For this review, take the finished solid that the model builds, in its own axes (mm). A direction names the side the tool comes from. Coordinates: 2 decimals unless noted, no trailing zeros.
```python
from build123d import *

# Parameters (mm, degrees)
BOSS_EXTRUDE1_DEPTH = 0.7
SCALE1_SCALE        = 3


with BuildPart() as part:
    # Sketch1 → Boss-Extrude1 (new body)
    with BuildSketch(Plane.XY):
        with BuildLine():
            add(Edge.make_bspline(
                [(1.308612852, 4.749134037), (1.089185384, 3.585197579), (1.793550911, 2.587518606)],
                knots=[0, 0, 0, 1, 1, 1], degree=2))
            ThreePointArc((1.793550911, 2.587518606), (1.734959229, -0.853049688), (-1.670369344, -0.358397807))
            Line((-1.670369344, -0.358397807), (1.14, -0.358397807))
            Line((1.14, -0.358397807), (1.14, 0))
            Line((1.14, 0), (0.84, 0))
            Line((0.84, 0), (0.84, 0.615282796))
            Line((0.84, 0.615282796), (0.34, 0.615282796))
            Line((0.34, 0.615282796), (0.34, 0))
            Line((0.34, 0), (0, 0))
            Line((0, 0), (0, 0.615282796))
            Line((0, 0.615282796), (-0.5, 0.615282796))
            Line((-0.5, 0.615282796), (-0.5, 0.015282796))
            Line((-0.5, 0.015282796), (-1.86741437, 0.015282796))
            add(Edge.make_bspline(
                [(-1.86741437, 0.015282796), (-1.967195235, 0.235858372), (-2.024440964, 0.467418027), (-2.039152584, 0.709940467)],
                knots=[0, 0, 0, 0, 0.800781106, 0.800781106, 0.800781106, 0.800781106], degree=3))
            add(Edge.make_bspline(
                [(-2.039152584, 0.709940467), (-2.047148733, 0.925627975), (-2.02218467, 1.604112941), (-1.789435207, 2.864813182), (-0.855181509, 3.674882666), (-0.25, 3.615282796)],
                knots=[0.156243254, 0.156243254, 0.156243254, 0.156243254, 0.300823298, 0.609121374, 1, 1, 1, 1], degree=3))
            add(Edge.make_bspline(
                [(-0.25, 3.615282796), (-0.677964438, 3.343186963), (-0.807483326, 2.788196328), (-0.75, 2.315282796)],
                knots=[0, 0, 0, 0, 1, 1, 1, 1], degree=3))
            ThreePointArc((-0.75, 2.315282796), (-0.25, 1.815282796), (0.25, 2.315282796))
            add(Edge.make_bspline(
                [(0.25, 2.315282796), (0.215460935, 2.756941027), (0.29493392, 3.342860109), (0.442449357, 4.258464168), (0.878924002, 4.555096789), (1.14, 4.675619868)],
                knots=[0, 0, 0, 0, 0.483638441, 0.672292201, 1, 1, 1, 1], degree=3))
            add(Edge.make_bspline(
                [(1.14, 4.675619868), (1.224306426, 4.712376952), (1.308612852, 4.749134037)],
                knots=[0, 0, 0, 0.865241942, 0.865241942, 0.865241942], degree=2))
        make_face()
    extrude(amount=BOSS_EXTRUDE1_DEPTH)


with BuildPart() as part_1:
    # Scale1: scaled about (0.30944177, 1.215178074, 0.35)
    add(part.part.scale(SCALE1_SCALE).moved(Location((-0.61888354, -2.430356148, -0.7))))


solid = part_1.part
```
1) Consider section A-A (x = -1.75). Count the separate pieces of the cut face and the enclosed holes in it, then the cut area to 3 significant figures.
2) Clearance check with flat-ended pins moving along their axes: P1, Ø1, axis at y = 5, z = -0.5, coming from the +X side; P2, Ø1, axis at x = 2.5, z = 0, coming from the -Y side; P3, Ø0.9, axis at y = -1.5, z = 0.5, coming from the -X side. State where each tip first meets the part, or that it passes through.
3) Tool access review of faces 4 (the face through (2.4, -2.43, 0.3)), 5 (the face through (0, 1, -0.7)), 6 (the face through (-2.119, -1, 0)): name each direction out of +Z, -Z, +X, -X, +Y, -Y from which nothing blocks a thin tool from reaching the whole face with its end or side.
4) For L1, parallel to Y at x = -1.25, z = 0.6; L2, parallel to X at y = 0.5, z = -0.15; L3, parallel to X at y = 6.5, z = 1.35, list the stretches that pass through material, from the lowest coordinate up.
5) The part is to be moulded in two halves that separate along Y. For faces 1 (the face through (0, 1, 1.4)), 2 (the face through (-0.619, -2, 0)), 3 (the face through (4.71, -4.88, 0.34)), say which applies: pulls with the +Y half, pulls with the -Y half, needs draft (parallel to the pull), parting line crosses it, or undercut.
Results:
1. separate pieces: 3
1. enclosed holes: 0
1. area: 14.3 mm2
2. P1: stops at x = 5.54
2. P2: stops at y = -6.37
2. P3: stops at x = -6.64
3. face 4: +Z, -Z, -X
3. face 5: -Z, +X, -X, +Y, -Y
3. face 6: +Z, -Z
4. L1: y = -6.49 to -3.51, -0.58 to 3.02
4. L2: x = -6.74 to 7
4. L3: x = -5.07 to -2.72, 0.15 to 4.05
5. face 1: needs draft
5. face 2: undercut
5. face 3: parting line crosses it
